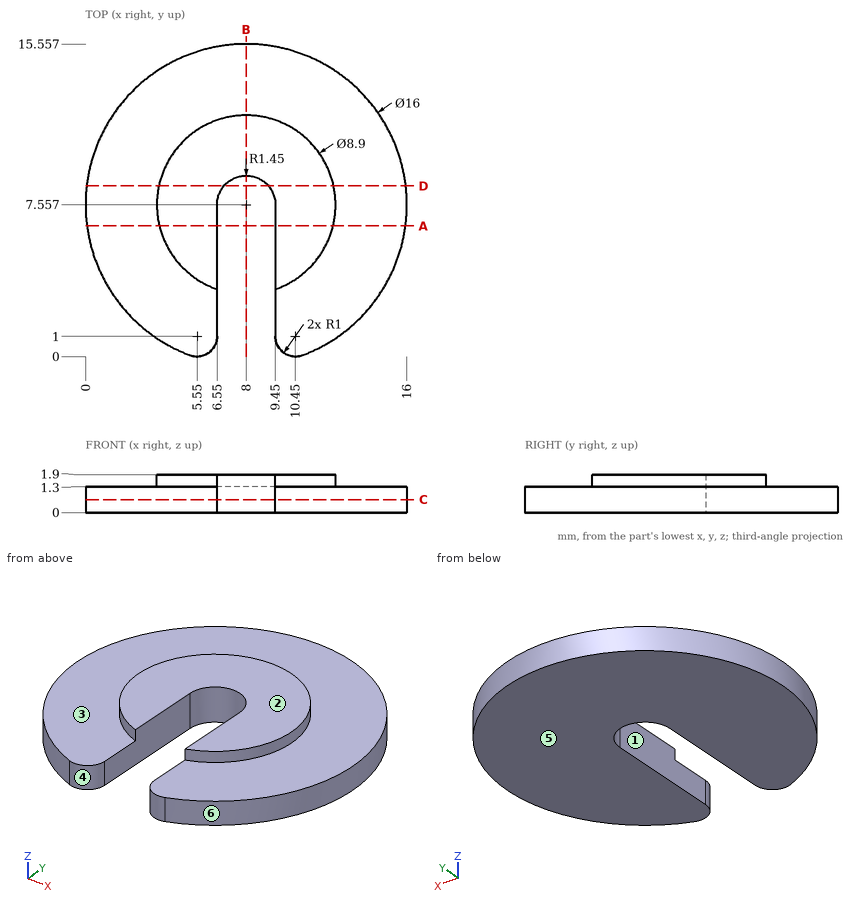
Drawing for the job (mm, zero at the part's lowest x, y, z). A direction names the side the tool comes from. Round coordinates to 2 decimals unless told otherwise and drop trailing zeros. Write each loop counter-clockwise with the first axis right and the second up, starting at its lowest first coordinate (ties: lowest second). Pieces come first, ordered by that corner, then holes. Notation, with made-up numbers: M 27,-23.75 L 31,-23.75 A20 ccw 31,15.25 Z; hole C 18,17 d9. An arc over 180 degrees is marked long. Answer as a JSON object with one key per item and string values. Group by question number.
(1) Cut at B-B (x = 8). Give the cut face in (y, z).
(2) Cut at D-D (y = 8.5). Give the cut face in (x, z).
(3) Cut at C-C (z = 0.65). Give the cut face in (x, y).
(4) Drill centre lines: L1, parallel to X at y = 7.5, z = 1.15; L2, parallel to Z at x = 4, y = 13; L3, parallel to X at y = 8.5, z = 0.45 (1 decimal). Where is each one in solid material? Low to high.
(5) Cut at A-A (y = 6.5). Give the cut face in (x, z).
(6) Flat gauge pins, fed straight in: pin 1 (1 mm diameter, centred on x = 13, z = 1, fed in from +Y); pin 2 (2 mm diameter, centred on x = 2, y = 6, fed in from +Z); pin 3 (0.6 mm diameter, centred on y = 3, z = 0.5, fed in from +X). Where does each tip first touch, or does it go through?
(7) Mould opens along X. For the marked faces 4, 5 and 6 say: pulls with the +X half, pulls with the -X half, needs draft (parallel to the pull), parting line crosses it, or undercut.
(8) Which spindle directions (+Z, -Z, +X, -X, +Y, -Y) get a long thin tool onto all of the face, cutting with end or side? Do the marked faces 1, 2 and 3. Say none if no direction does.
Responses:
{
 "1": {"outline": "M 9.01,0 L 15.56,0 L 15.56,1.3 L 12.01,1.3 L 12.01,1.9 L 9.01,1.9 Z"},
 "2": {"outline": "M 0.06,0 L 6.9,0 L 6.9,1.9 L 3.65,1.9 L 3.65,1.3 L 0.06,1.3 Z; M 9.1,0 L 15.94,0 L 15.94,1.3 L 12.35,1.3 L 12.35,1.9 L 9.1,1.9 Z"},
 "3": {"outline": "M 5.2,0.06 A1 ccw 6.55,1 L 6.55,7.56 A1.45 cw 9.45,7.56 L 9.45,1 A1 ccw 10.8,0.06 A8 ccw long Z"},
 "4": {"L1": "x = 0 to 6.55, 9.45 to 16", "L2": "z = 0 to 1.3", "L3": "x = 0.1 to 6.9, 9.1 to 15.9"},
 "5": {"outline": "M 0.07,0 L 6.55,0 L 6.55,1.9 L 3.68,1.9 L 3.68,1.3 L 0.07,1.3 Z; M 9.45,0 L 15.93,0 L 15.93,1.3 L 12.32,1.3 L 12.32,1.9 L 9.45,1.9 Z"},
 "6": {"pin 1": "stops at y = 14.17", "pin 2": "stops at z = 1.3", "pin 3": "stops at x = 14.77"},
 "7": {"face 4": "undercut", "face 5": "needs draft", "face 6": "parting line crosses it"},
 "8": {"face 1": "+Z, -Z, -Y", "face 2": "+Z, +X, -X, +Y, -Y", "face 3": "+Z"}
}
